Read the model definition and answer for the solid it produces. Units are mm, in the model's axes. Face numbers are marked on the shaded views. A direction names the side the tool comes from. Give positions to 0.01 mm unless a question says otherwise; leave off trailing zeros. Order: outer loops, then holes, each group sorted by start corner. A loop starts at its lowest first (then second) coordinate and runs counter-clockwise, first axis right, second up. Notation, with made-up numbers: (9.25, 11) -> (18.25, 11) arc R22 ccw to (18.25, 32) -> close; hole circle Ø8 at (-11.75, 56.25). An arc over 180 degrees is marked (long way). Answer as CSV lines item,"result". Start each with the question number.
1) Find section C-C (z = 63.5). Determine the outline of the cut face in (x, y).
2) Find section D-D (x = 361). Determine the outline of the cut face in (y, z), and give its area (3 significant figures).
3) Flat-ended cylindrical pins translate along their axes: pin 1 Ø3.5 at (x, y) = (483, 42) entering from -Z; pin 2 Ø8 at (x, y) = (451.5, 40.5) entering from +Z; pin 3 Ø4 at (y, z) = (51.5, -39) entering from -X. Find the tip coordinate at first contact, or state that the pin passes through.
4) Find section B-B (x = 42). Determine the outline of the cut face in (y, z), and give its area (3 significant figures).
5) Straight lines are drawn through the part: L1, parallel to X at y = -67, z = -29; L2, parallel to X at y = 24, z = -57; L3, parallel to Z at x = 299, y = 21. For each, find the intervals that lie inside material, in ascending order. Write a range as from..to.
6) For the marked faces 1, 2 and 3, determine the directions among +Z, -Z, +X, -X, +Y, -Y from which every point of the face is accessible in a straight line to the end or side of a thin tool.
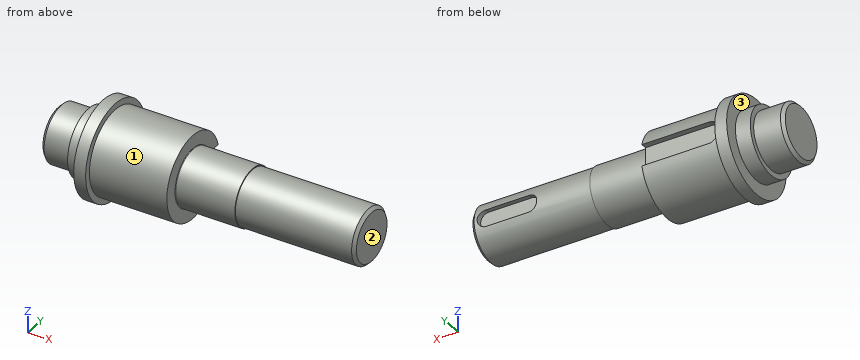
```python
from build123d import *

# Parameters (mm, degrees)
CUT_EXTRUDE_1_DEPTH = 12
CUT_EXTRUDE_START   = 36.5
CUT_EXTRUDE_2_DEPTH = 501.552138996
CHAMFER_1_SIZE      = 5
FILLET_1_R          = 1


with BuildPart() as part:
    # 草图1 → 旋转1 (revolve)
    with BuildSketch(Plane.XY, mode=Mode.PRIVATE) as revolve_1_sk:
        Polygon((0, 0), (0, 47.5), (50, 47.5), (50, 56.5), (75, 56.5), (75, 80), (95, 80), (95, 70), (225, 70), (225, 47.5), (325, 47.5), (325, 46), (525, 46), (525, 0), align=None)
    revolve(revolve_1_sk.sketch.rotate(Axis((0, 0, 0), (1, 0, 0)), 90), axis=Axis((0, 0, 0), (1, 0, 0)))

    # 草图2 → 切除-拉伸1 (cut)
    with BuildSketch(Plane(origin=(0, 70, 0), x_dir=(-1, 0, 0), z_dir=(0, 1, 0))):
        with BuildLine():
            Line((-225, 18), (-225, -18))
            Line((-225, -18), (-113, -18))
            ThreePointArc((-113, -18), (-95, 0), (-113, 18))
            Line((-113, 18), (-225, 18))
        make_face()
    extrude(amount=-CUT_EXTRUDE_1_DEPTH, mode=Mode.SUBTRACT)

    # 草图3 → 切除-拉伸2 (cut, through all)
    with BuildSketch(Plane(origin=(0, 0, 0), x_dir=(-1, 0, 0), z_dir=(0, 1, 0)).offset(CUT_EXTRUDE_START)):
        with BuildLine():
            Line((-429, 14), (-501, 14))
            ThreePointArc((-501, 14), (-515, 0), (-501, -14))
            Line((-501, -14), (-429, -14))
            ThreePointArc((-429, -14), (-415, 0), (-429, 14))
        make_face()
    extrude(amount=CUT_EXTRUDE_2_DEPTH, mode=Mode.SUBTRACT)

    # 倒角1
    chamfer_1_edges = [part.edges().sort_by_distance(p)[0] for p in [
        (0, 0, -47.5),
        (525, 0, -46),
    ]]
    chamfer(chamfer_1_edges, length=CHAMFER_1_SIZE)

    # 圆角1
    fillet_1_edges = [part.edges().sort_by_distance(p)[0] for p in [
        (225, 0, -47.5),
    ]]
    fillet(fillet_1_edges, radius=FILLET_1_R)


solid = part.part
```
Findings below:
1,outline,"(75, -48.66) -> (95, -48.66) -> (95, -29.46) -> (225, -29.46) -> (225, 29.46) -> (95, 29.46) -> (95, 48.66) -> (75, 48.66) -> close"
2,outline,"circle Ø92 at (0, 0)"
2,area,"6,650 mm²"
3,pin 1,"z = -22.27"
3,pin 2,"z = 28"
3,pin 3,"x = 75"
4,outline,"circle Ø95 at (0, 0)"
4,area,"7,090 mm²"
5,L1,"75..95"
5,L2,"75..225"
5,L3,"-42.61..42.61"
6,face 1,"+X"
6,face 2,"+Z, -Z, +X, +Y, -Y"
6,face 3,"-X"
